Geometry: final body of the model. Coordinates: model frame, mm. Face numbers are marked on the shaded views. A direction names the side the tool comes from. Give positions to 0.01 mm unless a question says otherwise; leave off trailing zeros. Order: outer loops, then holes, each group sorted by start corner. A loop starts at its lowest first (then second) coordinate and runs counter-clockwise, first axis right, second up. Notation, with made-up numbers: M 82,84 L 119,84 A20 ccw 119,104 Z; hole C 59.5,75.25 d2. An arc over 180 degrees is marked long. Use CSV: the item, a comma, the result in double quotes.
```python
from build123d import *

# Parameters (mm, degrees)
PAD_DEPTH       = 8
SKETCH001_W     = 8
SKETCH001_H     = 9.5
SKETCH001_H_2   = 24
SKETCH001_W_2   = 7.7
SKETCH001_H_3   = 8
POCKET_DEPTH    = 9
SKETCH002_R     = 1.7
POCKET001_DEPTH = 9
SKETCH003_R     = 1.7
POCKET002_DEPTH = 35


with BuildPart() as part:
    # Sketch → Pad (new body)
    with BuildSketch(Plane.XY):
        Polygon((0, 0), (-34.6, 0), (-34.6, 40.6), (-25, 40.6), (-25, 9.6), (0, 9.6), align=None)
    extrude(amount=PAD_DEPTH)

    # Sketch001 → Pocket (cut)
    with BuildSketch(Plane.XY.offset(8)):
        with Locations((-30.6, 35.85)):
            Rectangle(SKETCH001_W, SKETCH001_H)
        with Locations((-30.6, 12)):
            Rectangle(SKETCH001_W, SKETCH001_H_2)
        with Locations((-8.15, 5.6)):
            Rectangle(SKETCH001_W_2, SKETCH001_H_3)
    extrude(amount=-POCKET_DEPTH, mode=Mode.SUBTRACT)

    # Sketch002 → Pocket001 (cut)
    with BuildSketch(Plane.XZ.offset(-24)):
        with Locations((-30, 4)):
            Circle(SKETCH002_R)
    extrude(amount=-POCKET001_DEPTH, mode=Mode.SUBTRACT)

    # Sketch003 → Pocket002 (cut)
    with BuildSketch(Plane.YZ):
        with Locations((5, 4)):
            Circle(SKETCH003_R)
    extrude(amount=-POCKET002_DEPTH, mode=Mode.SUBTRACT)


solid = part.part
```
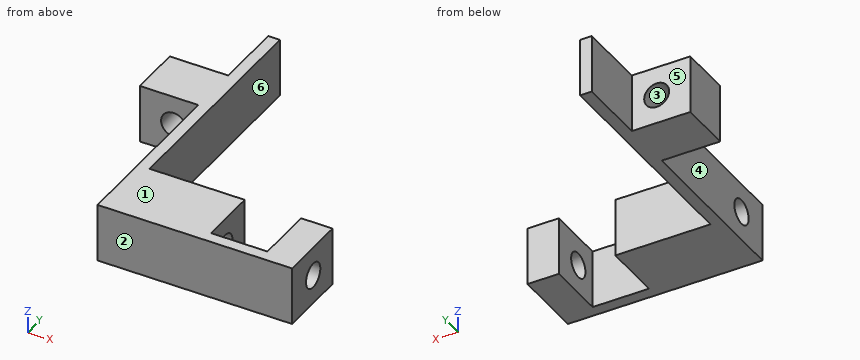
1. Section A-A, the plane y = 5. Return the cut outline in (x, z), plus the area to 3 significant figures.
Answer:
outline,"M -26.6,0 L -12,0 L -12,2.3 L -26.6,2.3 Z; M -26.6,5.7 L -12,5.7 L -12,8 L -26.6,8 Z; M -4.3,0 L 0,0 L 0,2.3 L -4.3,2.3 Z; M -4.3,5.7 L 0,5.7 L 0,8 L -4.3,8 Z"
area,"86.9 mm2"
2. Section C-C, the plane x = -30. Return the cut outline in (y, z).
Answer:
outline,"M 24,0 L 31.1,0 L 31.1,2.3 L 24,2.3 Z; M 24,5.7 L 31.1,5.7 L 31.1,8 L 24,8 Z"
3. Section B-B, the plane z = 4. Return the cut outline in (x, y), plus the area to 3 significant figures.
Answer:
outline,"M -34.6,24 L -31.7,24 L -31.7,31.1 L -34.6,31.1 Z; M -28.3,24 L -26.6,24 L -26.6,6.7 L -12,6.7 L -12,9.6 L -25,9.6 L -25,40.6 L -26.6,40.6 L -26.6,31.1 L -28.3,31.1 Z; M -26.6,0 L 0,0 L 0,3.3 L -4.3,3.3 L -4.3,1.6 L -12,1.6 L -12,3.3 L -26.6,3.3 Z; M -4.3,6.7 L 0,6.7 L 0,9.6 L -4.3,9.6 Z"
area,"212 mm2"
4. Reachability of the marked faces 4, 5 and 6 from +Z, -Z, +X, -X, +Y, -Y: full face, straight path, thin tool, end or side. Return the list, or none.
Answer:
face 4,"+Z, -Z, -X, -Y"
face 5,"+Z, -Z, -X, +Y"
face 6,"+Z, -Z, +X, +Y"
5. Pull-direction query (Z, two-part tool) for the marked faces 1, 2 and 3; classes: +Z half, -Z half, draft (parallel to the pull), parting line (faces both ways), or undercut.
Answer:
face 1,"+Z half"
face 2,"draft"
face 3,"undercut"
6. Pin query (flat end, axial travel): pin 1 Ø4 at (x, z) = (-21.5, 2) entering from +Y; pin 2 Ø2.5 at (y, z) = (33, 5.5) entering from +X; pin 3 Ø3 at (y, z) = (5, 4) entering from +X; pin 4 Ø4 at (x, z) = (-32, 5) entering from -Y. Return the tip coordinate at first contact, or that it passes through.
Answer:
pin 1,"y = 9.6"
pin 2,"x = -25"
pin 3,"through"
pin 4,"y = 24"
7. Section D-D, the plane x = -26. Return the cut outline in (y, z).
Answer:
outline,"M 0,0 L 40.6,0 L 40.6,8 L 0,8 Z; hole C 5,4 d3.4"
8. Line query: line 1 (Z direction, x = -1.2, y = 5); line 2 (X direction, y = 4, z = 5.75); line 3 (X direction, y = 15.5, z = 3). Output: solid intervals per line, ascending.
Answer:
line 1,"0 to 2.3, 5.7 to 8"
line 2,"-26.6 to -12, -4.3 to 0"
line 3,"-26.6 to -25"
